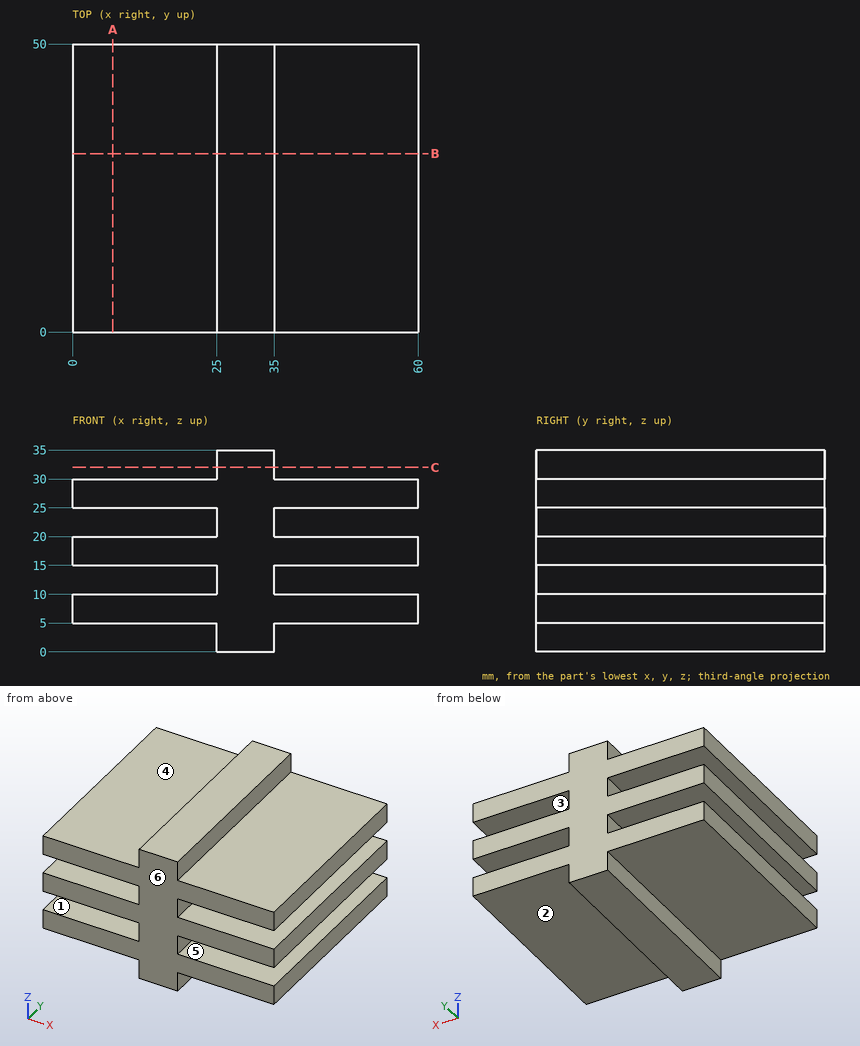
Check sheet for the drawn part. Datum: minimum x, y, z corner. Units: mm. A direction names the side the tool comes from. Round coordinates to 2 decimals unless told otherwise and drop trailing zeros. Order: outer loops, then holes, each group sorted by start corner. A loop starts at its lowest first (then second) coordinate and runs counter-clockwise, first axis right, second up. Notation, with made-up numbers: M -11,70 L 39,70 A29 cw 39,108 Z; hole C -15,28 d5. An arc over 180 degrees is marked long. Answer in a Markdown table with one row per item.
(1) Gauge pin test, flat ends, axial feed: pin 1 (2.5 mm diameter, centred on y = 20, z = 32.5, fed in from +X); pin 2 (1.5 mm diameter, centred on y = 26, z = 22, fed in from -X); pin 3 (5.5 mm diameter, centred on y = 32, z = 2.5, fed in from -X); pin 4 (20 mm diameter, centred on x = 51.5, y = 33.5, fed in from -Z). Record the tip position at first contact, or that the pin passes through.
Findings:
| item | result |
|---|---|
| pin 1 | stops at x = 35 |
| pin 2 | stops at x = 25 |
| pin 3 | stops at x = 0 |
| pin 4 | stops at z = 5 |
(2) Section check C-C on z = 32. Record the boundary of the cut face in (x, y).
Findings:
| item | result |
|---|---|
| outline | M 25,0 L 35,0 L 35,50 L 25,50 Z |
(3) Section check B-B on y = 31. Record the boundary of the cut face in (x, z), plus the area to 3 significant figures.
Findings:
| item | result |
|---|---|
| outline | M 0,5 L 25,5 L 25,0 L 35,0 L 35,5 L 60,5 L 60,10 L 35,10 L 35,15 L 60,15 L 60,20 L 35,20 L 35,25 L 60,25 L 60,30 L 35,30 L 35,35 L 25,35 L 25,30 L 0,30 L 0,25 L 25,25 L 25,20 L 0,20 L 0,15 L 25,15 L 25,10 L 0,10 Z |
| area | 1,100 mm^2 |
(4) Draft check along Z on the marked faces 4, 5 and 6. Enter one of: +Z half, -Z half, draft (parallel to the pull), parting line (faces both ways), or undercut.
Findings:
| item | result |
|---|---|
| face 4 | +Z half |
| face 5 | undercut |
| face 6 | draft |
(5) Set-up check for the marked faces 1, 2 and 3: record each of +Z, -Z, +X, -X, +Y, -Y from which the full face is reachable in a straight line by a thin tool's end or side.
Findings:
| item | result |
|---|---|
| face 1 | -X, +Y, -Y |
| face 2 | -Z, +X, +Y, -Y |
| face 3 | +X, +Y, -Y |
(6) Section check A-A on x = 7. Record the boundary of the cut face in (y, z).
Findings:
| item | result |
|---|---|
| outline | M 0,5 L 50,5 L 50,10 L 0,10 Z; M 0,15 L 50,15 L 50,20 L 0,20 Z; M 0,25 L 50,25 L 50,30 L 0,30 Z |
(7) Material ranges on line 1 along Z through (x, y) = (56, 41); line 2 along X through (y, z) = (21, 22), recorded low to high. Write a range as from..to.
Findings:
| item | result |
|---|---|
| line 1 | z = 5..10, 15..20, 25..30 |
| line 2 | x = 25..35 |
